Work out the finished part from the listing and answer in its coordinate system (mm). A direction names the side the tool comes from. Coordinates: 2 decimals unless noted, no trailing zeros. Order: outer loops, then holes, each group sorted by start corner. A loop starts at its lowest first (then second) coordinate and runs counter-clockwise, first axis right, second up.
```python
from build123d import *

# Parameters (mm, degrees)
SKETCH1_W           = 740.664
SKETCH1_H           = 914.4
BOSS_EXTRUDE1_DEPTH = 203.2
SHELL1_T            = -6.35
SKETCH4_R           = 25.4
CUT_EXTRUDE1_DEPTH  = 853.694
FILLET1_R           = 38.1
SCALE1_SCALE        = 0.5867


with BuildPart() as part:
    # Sketch1 → Boss-Extrude1 (new body)
    with BuildSketch(Plane(origin=(0, 0, 0), x_dir=(0, 0, -1), z_dir=(1, 0, 0))):
        Rectangle(SKETCH1_W, SKETCH1_H)
    extrude(amount=BOSS_EXTRUDE1_DEPTH)

    # Shell1
    shell1_openings = [part.faces().sort_by_distance(p)[0] for p in [
        (0, 0, 0),
    ]]
    offset(amount=SHELL1_T, openings=shell1_openings, kind=Kind.INTERSECTION)

    # Sketch4 → Cut-Extrude1 (cut)
    with BuildSketch(Plane.XY.offset(370.332)):
        with Locations((103.042772695, 378.994204807)):
            Circle(SKETCH4_R)
    cut_extrude1 = extrude(amount=-CUT_EXTRUDE1_DEPTH, mode=Mode.SUBTRACT)

    # Mirror1: Cut-Extrude1 across plane
    add(cut_extrude1.mirror(Plane.ZX), mode=Mode.SUBTRACT)

    # Fillet1
    fillet1_edges = [part.edges().sort_by_distance(p)[0] for p in [
        (203.2, -457.2, 0),
    ]]
    fillet(fillet1_edges, radius=FILLET1_R)
    fillet1_2_edges = [part.edges().sort_by_distance(p)[0] for p in [
        (203.2, 457.2, 0),
    ]]
    fillet(fillet1_2_edges, radius=FILLET1_R)
    # the kernel refuses this fillet: 38.1 mm, written as the material it takes off along each edge
    with BuildSketch(Plane(origin=(0, -457.2, -465.582), x_dir=(1, 0, 0), z_dir=(0, 0, 1))) as fillet1_3_piece_1:
        with BuildLine():
            CenterArc((FILLET1_R, FILLET1_R), FILLET1_R, 180, 90)
            Line((0, FILLET1_R), (-FILLET1_R * 0.02, FILLET1_R))
            Line((-FILLET1_R * 0.02, FILLET1_R), (-FILLET1_R * 0.02, -FILLET1_R * 0.02))
            Line((-FILLET1_R * 0.02, -FILLET1_R * 0.02), (FILLET1_R, -FILLET1_R * 0.02))
            Line((FILLET1_R, -FILLET1_R * 0.02), (FILLET1_R, 0))
        make_face()
    extrude(amount=931.164, mode=Mode.SUBTRACT)
    # the kernel refuses this fillet: 38.1 mm, written as the material it takes off along each edge
    with BuildSketch(Plane(origin=(0, 457.2, 465.582), x_dir=(1, 0, 0), z_dir=(0, 0, -1))) as fillet1_4_piece_1:
        with BuildLine():
            CenterArc((FILLET1_R, FILLET1_R), FILLET1_R, 180, 90)
            Line((0, FILLET1_R), (-FILLET1_R * 0.02, FILLET1_R))
            Line((-FILLET1_R * 0.02, FILLET1_R), (-FILLET1_R * 0.02, -FILLET1_R * 0.02))
            Line((-FILLET1_R * 0.02, -FILLET1_R * 0.02), (FILLET1_R, -FILLET1_R * 0.02))
            Line((FILLET1_R, -FILLET1_R * 0.02), (FILLET1_R, 0))
        make_face()
    extrude(amount=931.164, mode=Mode.SUBTRACT)


with BuildPart() as part_1:
    # Scale1: scaled about (152.162233958, 0, 0)
    add(part.part.scale(SCALE1_SCALE).moved(Location((62.888651295, 0, 0))))


solid = part_1.part
```
1. For faces 1 (the cylindrical face through (175.73, 261.52, -3.04)), 2 (the flat face through (120, -4, -213.548)), 3 (the cylindrical face through (121.4, -237.13, 215.44)), determine the directions among +Z, -Z, +X, -X, +Y, -Y from which every point of the face is accessible in a straight line to the end or side of a thin tool.
2. Consider probe 1 along Z at (x, y) = (69, 91); probe 2 along Y at (x, z) = (159, 193); probe 3 along X at (y, z) = (73.5, -159.5). Determine where each line is inside the solid, lowest interval first.
3. The mould has two halves that part along X. Classify faces 4 (the cylindrical face through (121.4, -237.13, -215.38)), 5 (the cylindrical face through (175.384, -261.865, -3.042)), 6 (the cylindrical face through (79.377, -267.456, -1.014)), 7 (the flat face through (122, -4, 217.274)): released by +X, released by -X, zero draft, split by the parting line, or undercut.
4. The part is cut by section D-D (y = -109). Determine the outline of the cut face in (x, z).
5. A flat-ended cylindrical pin translates along its axis: pin 1 (8 mm diameter, centred on y = -88.5, z = 4.5, fed in from -X). Find the tip coordinate at first contact, or state that the pin passes through.
6. The part is cut by section C-C (x = 120). Determine the outline of the cut face in (y, z), plus the area to 3 significant figures.
7. The part is cut by section A-A (x = 152). Determine the outline of the cut face in (y, z).
Worked out:
1. face 1: none
1. face 2: -X
1. face 3: +Z, -Z
2. probe 1: z = -217.27 to -213.55, 213.55 to 217.27
2. probe 2: y = -268.24 to -264.51, 264.51 to 268.24
2. probe 3: x = 178.38 to 182.11
3. face 4: undercut
3. face 5: undercut
3. face 6: released by -X
3. face 7: zero draft
4. outline: (62.89, -217.27) - (182.11, -217.27) - (182.11, 217.27) - (62.89, 217.27) - (62.89, 213.55) - (178.38, 213.55) - (178.38, -213.55) - (62.89, -213.55) - close
5. pin 1: stops at x = 178.38
6. outline: (-268.24, -217.27) - (-236.88, -217.27) - (-236.88, -213.55) - (-264.51, -213.55) - (-264.51, 213.55) - (-236.88, 213.55) - (-236.88, 217.27) - (-268.24, 217.27) - close; (-207.83, -217.27) - (207.83, -217.27) - (207.83, -213.55) - (-207.83, -213.55) - close; (-207.83, 213.55) - (207.83, 213.55) - (207.83, 217.27) - (-207.83, 217.27) - close; (236.88, -217.27) - (268.24, -217.27) - (268.24, 217.27) - (236.88, 217.27) - (236.88, 213.55) - (264.51, 213.55) - (264.51, -213.55) - (236.88, -213.55) - close
6. area: 6,750 mm2
7. outline: (-268.24, -217.27) - (268.24, -217.27) - (268.24, 217.27) - (-268.24, 217.27) - close; hole (-264.51, -213.55) - (264.51, -213.55) - (264.51, 213.55) - (-264.51, 213.55) - close
